from build123d import *

# Parameters (mm, degrees)
SKETCH1_R           = 25.4
BOSS_EXTRUDE1_DEPTH = 10
SKETCH2_R           = 29.9
BOSS_EXTRUDE2_DEPTH = 5
SKETCH3_R           = 3
CUT_EXTRUDE1_DEPTH  = 76.628


with BuildPart() as part:
    # Sketch1 → Boss-Extrude1 (new body, symmetric)
    with BuildSketch(Plane.XY):
        Circle(SKETCH1_R)
    extrude(amount=BOSS_EXTRUDE1_DEPTH, both=True)

    # Sketch2 → Boss-Extrude2 (add)
    with BuildSketch(Plane.XY.offset(10)):
        Circle(SKETCH2_R)
    boss_extrude2 = extrude(amount=BOSS_EXTRUDE2_DEPTH)

    # Mirror1: Boss-Extrude2 across plane
    add(boss_extrude2.mirror(Plane.XY))

    # Sketch3 → Cut-Extrude1 (cut)
    with BuildSketch(Plane.XY.offset(15)):
        Circle(SKETCH3_R)
    extrude(amount=-CUT_EXTRUDE1_DEPTH, mode=Mode.SUBTRACT)


solid = part.part
Verification items for the finished model (mm, model axes). A direction names the side the tool comes from. Give positions to 0.01 mm unless a question says otherwise; leave off trailing zeros. Loops run counter-clockwise (first coordinate to the right, second up) from the corner with the lowest first, then second, coordinate; pieces in that order, holes last.
1) Sectioned sample at A-A, the plane y = 0. Enter the section's corners in (x, z), then the cut area to 3 significant figures.
2) Set-up check for faces 4 (the flat face through (0, -6, -15)), 5 (the cylindrical face through (-5.506, -24.796, 0.14)): record each of +Z, -Z, +X, -X, +Y, -Y from which the full face is reachable in a straight line by a thin tool's end or side.
3) Depth check by flat-ended pin: pin 1 Ø8 at (x, z) = (21, -4.5) entering from +Y; pin 2 Ø8 at (x, z) = (-10, -0.5) entering from -Y; pin 3 Ø10 at (x, z) = (16.5, -2) entering from +Y. Enter the tip coordinate at first touch or a pass-through.
4) Draft check along Z on faces 1 (the cylindrical face through (13.797, -26.526, -12.465)), 2 (the flat face through (0, -6, 15)), 3 (the flat face through (-13, -22, -10)). Enter one of: pulls with the +Z half, pulls with the -Z half, needs draft (parallel to the pull), parting line crosses it, or undercut.
5) Thickness scan on line 1 along Y through (x, z) = (0, 7.5); line 2 along Z through (x, y) = (-22, -16.5); line 3 along Y through (x, z) = (2.5, -7.75). Record the ranges inside material, lowest first.
6) Sectioned sample at D-D, the plane x = -12.5. Enter the section's corners in (y, z).
7) Sectioned sample at C-C, the plane z = 9. Enter the section's corners in (x, y), then the cut area to 3 significant figures.
Answers:
1. outline: (-29.9, -15) - (-3, -15) - (-3, 15) - (-29.9, 15) - (-29.9, 10) - (-25.4, 10) - (-25.4, -10) - (-29.9, -10) - close; (3, -15) - (29.9, -15) - (29.9, -10) - (25.4, -10) - (25.4, 10) - (29.9, 10) - (29.9, 15) - (3, 15) - close
1. area: 1,430 mm2
2. face 4: -Z, +X, -X, +Y, -Y
2. face 5: none
3. pin 1: stops at y = 18.87
3. pin 2: stops at y = -24.68
3. pin 3: stops at y = 22.65
4. face 1: needs draft
4. face 2: pulls with the +Z half
4. face 3: undercut
5. line 1: y = -25.4 to -3, 3 to 25.4
5. line 2: z = -15 to -10, 10 to 15
5. line 3: y = -25.28 to -1.66, 1.66 to 25.28
6. outline: (-27.16, -15) - (27.16, -15) - (27.16, -10) - (22.11, -10) - (22.11, 10) - (27.16, 10) - (27.16, 15) - (-27.16, 15) - (-27.16, 10) - (-22.11, 10) - (-22.11, -10) - (-27.16, -10) - close
7. outline: circle Ø50.8 at (0, 0); hole circle Ø6 at (0, 0)
7. area: 2,000 mm2
